```python
from build123d import *

# Parameters (mm, degrees)
SKETCH_W        = 106.6
SKETCH_H        = 40
PAD_DEPTH       = 180
SKETCH001_W     = 102.8
SKETCH001_H     = 176.2
POCKET_DEPTH    = 38.1
SKETCH002_W     = 102.8
SKETCH002_H     = 1.9
POCKET001_DEPTH = 38.1
SKETCH003_W     = 50
SKETCH003_H     = 40
POCKET002_DEPTH = 5
SKETCH004_W     = 22
SKETCH004_H     = 20
POCKET003_DEPTH = 5
SKETCH005_W     = 75
SKETCH005_H     = 22
POCKET004_DEPTH = 5
SKETCH006_R     = 4
SKETCH006_R_2   = 4.25
POCKET005_DEPTH = 5
CHAMFER_SIZE    = 5
CHAMFER001_SIZE = 5
SKETCH007_W     = 5
SKETCH007_H     = 10
POCKET006_DEPTH = 5
SKETCH008_W     = 5
SKETCH008_H     = 10
POCKET007_DEPTH = 5
SKETCH009_W     = 19.8
SKETCH009_H     = 10
POCKET008_DEPTH = 5
SKETCH010_W     = 40
SKETCH010_H     = 5
PAD001_DEPTH    = 5
CHAMFER002_SIZE = 3.099
CHAMFER003_SIZE = 3
SKETCH011_W     = 40
SKETCH011_H     = 5
PAD002_DEPTH    = 5
CHAMFER004_SIZE = 3.099
CHAMFER005_SIZE = 3
SKETCH012_W     = 3.5
SKETCH012_H     = 22
POCKET009_DEPTH = 5
SKETCH013_W     = 3.5
SKETCH013_H     = 22
POCKET010_DEPTH = 5


with BuildPart() as part:
    # Sketch → Pad (new body)
    with BuildSketch(Plane.XY):
        Rectangle(SKETCH_W, SKETCH_H)
    extrude(amount=PAD_DEPTH)

    # Sketch001 (on Face1 of Pad) → Pocket (cut)
    with BuildSketch(Plane(origin=(0, 20, 0), x_dir=(-1, 0, 0), z_dir=(0, 1, 0))):
        with Locations((0, 90)):
            Rectangle(SKETCH001_W, SKETCH001_H)
    extrude(amount=-POCKET_DEPTH, mode=Mode.SUBTRACT)

    # Sketch002 (on Face1 of Pocket) → Pocket001 (cut)
    with BuildSketch(Plane(origin=(0, 20, 0), x_dir=(-1, 0, 0), z_dir=(0, 1, 0))):
        with Locations((0, 0.95)):
            Rectangle(SKETCH002_W, SKETCH002_H)
    extrude(amount=-POCKET001_DEPTH, mode=Mode.SUBTRACT)

    # Sketch003 (on Face11 of Pocket001) → Pocket002 (cut)
    with BuildSketch(Plane.XZ.offset(20)):
        with Locations((0, 20)):
            Rectangle(SKETCH003_W, SKETCH003_H)
    extrude(amount=-POCKET002_DEPTH, mode=Mode.SUBTRACT)

    # Sketch004 (on Face9 of Pocket002) → Pocket003 (cut)
    with BuildSketch(Plane.YZ.offset(53.3)):
        with Locations((0, 57.78728)):
            Rectangle(SKETCH004_W, SKETCH004_H)
    extrude(amount=-POCKET003_DEPTH, mode=Mode.SUBTRACT)

    # Sketch005 (on Face10 of Pocket003) → Pocket004 (cut)
    with BuildSketch(Plane.XY.offset(180)):
        Rectangle(SKETCH005_W, SKETCH005_H)
    extrude(amount=-POCKET004_DEPTH, mode=Mode.SUBTRACT)

    # Sketch006 (on Face12 of Pocket004) → Pocket005 (cut)
    with BuildSketch(Plane.XZ.offset(20)):
        with Locations((39.85, 19.5)):
            Circle(SKETCH006_R)
        with Locations((39.85, 38.2)):
            Circle(SKETCH006_R_2)
    extrude(amount=-POCKET005_DEPTH, mode=Mode.SUBTRACT)

    # Chamfer
    chamfer_edges = [part.edges().sort_by_distance(p)[0] for p in [
        (-51.4, -18.1, 90),
        (-51.4, 0.95, 178.1),
        (0, -18.1, 178.1),
        (51.4, -18.1, 90),
        (51.4, 0.95, 178.1),
    ]]
    chamfer(chamfer_edges, length=CHAMFER_SIZE)

    # Chamfer001
    chamfer001_edges = [part.edges().sort_by_distance(p)[0] for p in [
        (53.3, -20, 90),
        (-53.3, -20, 90),
        (0, -20, 180),
        (53.3, 0, 180),
        (-53.3, 0, 180),
    ]]
    chamfer(chamfer001_edges, length=CHAMFER001_SIZE)

    # Sketch007 (on Face9 of Chamfer001) → Pocket006 (cut)
    with BuildSketch(Plane.YZ.offset(53.3)):
        with Locations((7.5, 145)):
            Rectangle(SKETCH007_W, SKETCH007_H)
        with Locations((7.5, 35)):
            Rectangle(SKETCH007_W, SKETCH007_H)
    extrude(amount=-POCKET006_DEPTH, mode=Mode.SUBTRACT)

    # Sketch008 (on Face2 of Pocket006) → Pocket007 (cut)
    with BuildSketch(Plane(origin=(-53.3, 0, 0), x_dir=(0, -1, 0), z_dir=(-1, 0, 0))):
        with Locations((-7.5, 145)):
            Rectangle(SKETCH008_W, SKETCH008_H)
        with Locations((-7.5, 35)):
            Rectangle(SKETCH008_W, SKETCH008_H)
    extrude(amount=-POCKET007_DEPTH, mode=Mode.SUBTRACT)

    # Sketch009 (on Face2 of Pocket007) → Pocket008 (cut)
    with BuildSketch(Plane(origin=(-53.3, 0, 0), x_dir=(0, -1, 0), z_dir=(-1, 0, 0))):
        with Locations((-10.1, 17.5)):
            Rectangle(SKETCH009_W, SKETCH009_H)
    extrude(amount=-POCKET008_DEPTH, mode=Mode.SUBTRACT)

    # Sketch010 (on Face4 of Pocket008) → Pad001 (join)
    with BuildSketch(Plane.YZ.offset(-51.4)):
        with Locations((0, 2.5)):
            Rectangle(SKETCH010_W, SKETCH010_H)
    extrude(amount=PAD001_DEPTH)

    # Chamfer002
    chamfer002_edges = [part.edges().sort_by_distance(p)[0] for p in [
        (-51.4, -20, 2.5),
    ]]
    chamfer(chamfer002_edges, length=CHAMFER002_SIZE)

    # Chamfer003
    chamfer003_edges = [part.edges().sort_by_distance(p)[0] for p in [
        (-46.4, 0.95, 5),
    ]]
    chamfer(chamfer003_edges, length=CHAMFER003_SIZE)

    # Sketch011 (on Face27 of Chamfer003) → Pad002 (join)
    with BuildSketch(Plane(origin=(51.4, 0, 0), x_dir=(0, -1, 0), z_dir=(-1, 0, 0))):
        with Locations((0, 2.5)):
            Rectangle(SKETCH011_W, SKETCH011_H)
    extrude(amount=PAD002_DEPTH)

    # Chamfer004
    chamfer004_edges = [part.edges().sort_by_distance(p)[0] for p in [
        (51.4, -20, 2.5),
    ]]
    chamfer(chamfer004_edges, length=CHAMFER004_SIZE)

    # Chamfer005
    chamfer005_edges = [part.edges().sort_by_distance(p)[0] for p in [
        (46.4, 0.95, 5),
    ]]
    chamfer(chamfer005_edges, length=CHAMFER005_SIZE)

    # Sketch012 (on Face15 of Chamfer005) → Pocket009 (cut)
    with BuildSketch(Plane.YZ.offset(53.3)):
        with Locations((18.25, 102)):
            Rectangle(SKETCH012_W, SKETCH012_H)
    extrude(amount=-POCKET009_DEPTH, mode=Mode.SUBTRACT)

    # Sketch013 (on Face52 of Pocket009) → Pocket010 (cut)
    with BuildSketch(Plane(origin=(-53.3, 0, 0), x_dir=(0, -1, 0), z_dir=(-1, 0, 0))):
        with Locations((-18.25, 102)):
            Rectangle(SKETCH013_W, SKETCH013_H)
    extrude(amount=-POCKET010_DEPTH, mode=Mode.SUBTRACT)


solid = part.part
```
Geometry: final body of the model. Coordinates: model frame, mm. A direction names the side the tool comes from. Give positions to 0.01 mm unless a question says otherwise; leave off trailing zeros. Loops run counter-clockwise (first coordinate to the right, second up) from the corner with the lowest first, then second, coordinate; pieces in that order, holes last. Notation, with made-up numbers: (37, 3.5) -> (56, 3.5) arc R18 cw to (56, 14.5) -> close; hole circle Ø3 at (6, -26). An arc over 180 degrees is marked (long way). Return JSON: item names as keys, results as strings.
Item 1: Section A-A, the plane z = 51. Output: boundary loops of the cut face in (x, y), plus the area to 3 significant figures.
Filled in:
{"outline": "(-53.3, -15) -> (-48.3, -20) -> (48.3, -20) -> (53.3, -15) -> (53.3, -11) -> (51.4, -11) -> (51.4, -13.1) -> (46.4, -18.1) -> (-46.4, -18.1) -> (-51.4, -13.1) -> (-51.4, 20) -> (-53.3, 20) -> close; (51.4, 11) -> (53.3, 11) -> (53.3, 20) -> (51.4, 20) -> close", "area": "306 mm^2"}
Item 2: Access query for faces 1 (the flat face through (48.9, -15.6, 86.4)), 2 (the flat face through (-50.8, -17.5, 86.3)), 3 (the flat face through (1, 15, 178.1)). Directions: +Z, -Z, +X, -X, +Y, -Y. A direction counts if a zero-diameter tool reaches every point of the face in a straight line with its end or side. Return the directions, or none.
Filled in:
{"face 1": "+Y", "face 2": "+Z, -Z, -X, -Y", "face 3": "-Z, +Y"}
Item 3: Pin query (flat end, axial travel): P1, Ø0.6, axis at x = 52.5, y = 8, coming from the -Z side; P2, Ø0.6, axis at x = -52, y = 19, coming from the +Z side; P3, Ø13.5, axis at x = 39.85, z = 38.2, coming from the +Y side; P4, Ø1.5, axis at x = 0.5, z = 179.5, coming from the -Y side. Return the tip coordinate at first contact, or that it passes through.
Filled in:
{"P1": "z = 0", "P2": "z = 176.6", "P3": "y = -17.9", "P4": "y = -16.25"}
Item 4: Section B-B, the plane y = -2.5. Output: boundary loops of the cut face in (x, z).
Filled in:
{"outline": "(-53.3, 0) -> (-46.4, 0) -> (-46.4, 2) -> (-49.4, 5) -> (-51.4, 5) -> (-51.4, 173.1) -> (-46.4, 178.1) -> (-37.5, 178.1) -> (-37.5, 180) -> (-48.3, 180) -> (-53.3, 175) -> close; (37.5, 178.1) -> (46.4, 178.1) -> (51.4, 173.1) -> (51.4, 67.79) -> (53.3, 67.79) -> (53.3, 175) -> (48.3, 180) -> (37.5, 180) -> close; (46.4, 0) -> (53.3, 0) -> (53.3, 47.79) -> (51.4, 47.79) -> (51.4, 5) -> (49.4, 5) -> (46.4, 2) -> close"}
Item 5: Mould query, pull axis Z, two halves, no side actions, for faces 4 (the flat face through (-1, 14, 180)), 5 (the flat face through (52, 20, 45)), 6 (the flat face through (-51.4, 4, 88)). Classes: released by +Z, released by -Z, zero draft, split by the parting line, or undercut.
Filled in:
{"face 4": "released by +Z", "face 5": "zero draft", "face 6": "undercut"}
Item 6: Section C-C, the plane x = 39.85. Output: boundary loops of the cut face in (y, z).
Filled in:
{"outline": "(-20, 0) -> (-18.1, 0) -> (-18.1, 15.5) -> (-20, 15.5) -> close; (-20, 23.5) -> (-18.1, 23.5) -> (-18.1, 33.95) -> (-20, 33.95) -> close; (-20, 42.45) -> (-18.1, 42.45) -> (-18.1, 173.1) -> (-13.1, 178.1) -> (20, 178.1) -> (20, 180) -> (-15, 180) -> (-20, 175) -> close"}
Item 7: Line query: line 1 (X direction, y = -19, z = 38); line 2 (X direction, y = 4, z = 93); line 3 (Z direction, x = 39, y = -19). Output: solid intervals per line, ascending.
Filled in:
{"line 1": "-49.3 to -25, 25 to 35.6, 44.1 to 49.3", "line 2": "-53.3 to -51.4, 51.4 to 53.3", "line 3": "0 to 15.59, 23.41 to 34.04, 42.36 to 176"}
Item 8: Section D-D, the plane z = 19.5. Output: boundary loops of the cut face in (x, y), plus the area to 4 significant figures.
Filled in:
{"outline": "(-53.3, -15) -> (-48.3, -20) -> (-25, -20) -> (-25, -18.1) -> (-46.4, -18.1) -> (-51.4, -13.1) -> (-51.4, 0.2) -> (-53.3, 0.2) -> close; (25, -20) -> (35.85, -20) -> (35.85, -18.1) -> (25, -18.1) -> close; (43.85, -20) -> (48.3, -20) -> (53.3, -15) -> (53.3, 20) -> (51.4, 20) -> (51.4, -13.1) -> (46.4, -18.1) -> (43.85, -18.1) -> close", "area": "199.5 mm^2"}
